from build123d import *

# Parameters (mm, degrees)
BOSS_EXTRUDE1_DEPTH = 3
SKETCH1_3_R         = 1.25
CUT_EXTRUDE1_DEPTH  = 3


with BuildPart() as part:
    # Sketch1 → Boss-Extrude1 (new body)
    with BuildSketch(Plane.XY):
        Polygon((-22.75, 9), (-12.75, 9), (12.75, 9), (22.75, 9), (22.75, -16), (12.75, -16), (12.75, 1), (-12.75, 1), (-12.75, -16), (-22.75, -16), align=None)
    extrude(amount=BOSS_EXTRUDE1_DEPTH)

    # Sketch1<3> → Cut-Extrude1 (cut)
    with BuildSketch(Plane.XY):
        with Locations((-16.25, -11)):
            Circle(SKETCH1_3_R)
        with Locations((16.25, -2)):
            Circle(SKETCH1_3_R)
        with Locations((16.25, -11)):
            Circle(SKETCH1_3_R)
        with Locations((-16.25, -2)):
            Circle(SKETCH1_3_R)
    extrude(amount=CUT_EXTRUDE1_DEPTH, mode=Mode.SUBTRACT)


solid = part.part
Work out the finished part from the listing and answer in its coordinate system (mm). A direction names the side the tool comes from. Round coordinates to 2 decimals unless told otherwise and drop trailing zeros. Write each loop counter-clockwise with the first axis right and the second up, starting at its lowest first coordinate (ties: lowest second). Pieces come first, ordered by that corner, then holes. Notation, with made-up numbers: (13.25, 75) -> (30.25, 75) arc R14 ccw to (30.25, 81) -> close; hole circle Ø10 at (66, 43.5). An arc over 180 degrees is marked (long way). Answer as CSV lines item,"result". Start each with the question number.
(1) Each of these flat-tipped pins is pushed along its axis until it touches: pin 1 (3 mm diameter, centred on x = -16.25, y = -2, fed in from -Z); pin 2 (2 mm diameter, centred on x = -16.25, y = -11, fed in from +Z). Where does it stop, or does it pass through?
(2) A tool of negligible diameter and unlimited length cuts with its end or side. For faces 1 (the cylindrical face through (-17.5, -1.95, 1.48)), 2 (the flat face through (12.75, -8, 1)), from which of +Z, -Z, +X, -X, +Y, -Y can it reach the whole face along a straight path? Write none if from no direction.
(3) Find the intervals of material crossed by probe 1 along Y at (x, z) = (-16.25, 1.2); probe 2 along X at (y, z) = (-6.5, 2.85); probe 3 along X at (y, z) = (-1, 0.95), in increasing order.
(4) The part is cut by section A-A, the plane y = -11. Give the vertices of the cut face in (x, z), then the cut area to 3 significant figures.
(5) The part is cut by section C-C, the plane z = 1.2. Give the vertices of the cut face in (x, y), then the cut area to 3 significant figures.
(6) The part is cut by section B-B, the plane x = -16.25. Give the vertices of the cut face in (y, z).
(7) The mould has two halves that part along Y. Classify faces 3 (the flat face through (0, 1, 1)), 4 (the flat face through (0, 9, 1)), 5 (the flat face through (-12.75, -7, 1)), 6 (the cylindrical face through (16.09, -9.76, 1.48)): +Y half, -Y half, draft (parallel to the pull), parting line (faces both ways), or undercut.
(8) The part is cut by section D-D, the plane x = 7. Give the vertices of the cut face in (y, z), then the cut area to 3 significant figures.
Output values:
1,pin 1,"stops at z = 0"
1,pin 2,"passes through"
2,face 1,"+Z, -Z"
2,face 2,"+Z, -Z, -Y"
3,probe 1,"y = -16 to -12.25, -9.75 to -3.25, -0.75 to 9"
3,probe 2,"x = -22.75 to -12.75, 12.75 to 22.75"
3,probe 3,"x = -22.75 to -17, -15.5 to -12.75, 12.75 to 15.5, 17 to 22.75"
4,outline,"(-22.75, 0) -> (-17.5, 0) -> (-17.5, 3) -> (-22.75, 3) -> close; (-15, 0) -> (-12.75, 0) -> (-12.75, 3) -> (-15, 3) -> close; (12.75, 0) -> (15, 0) -> (15, 3) -> (12.75, 3) -> close; (17.5, 0) -> (22.75, 0) -> (22.75, 3) -> (17.5, 3) -> close"
4,area,"45.0 mm²"
5,outline,"(-22.75, -16) -> (-12.75, -16) -> (-12.75, 1) -> (12.75, 1) -> (12.75, -16) -> (22.75, -16) -> (22.75, 9) -> (-22.75, 9) -> close; hole circle Ø2.5 at (-16.25, -11); hole circle Ø2.5 at (-16.25, -2); hole circle Ø2.5 at (16.25, -11); hole circle Ø2.5 at (16.25, -2)"
5,area,"684 mm²"
6,outline,"(-16, 0) -> (-12.25, 0) -> (-12.25, 3) -> (-16, 3) -> close; (-9.75, 0) -> (-3.25, 0) -> (-3.25, 3) -> (-9.75, 3) -> close; (-0.75, 0) -> (9, 0) -> (9, 3) -> (-0.75, 3) -> close"
7,face 3,"-Y half"
7,face 4,"+Y half"
7,face 5,"draft"
7,face 6,"undercut"
8,outline,"(1, 0) -> (9, 0) -> (9, 3) -> (1, 3) -> close"
8,area,"24.0 mm²"
